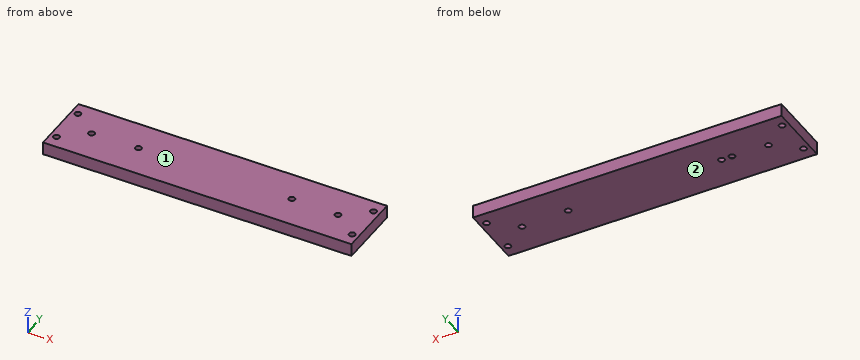
```python
from build123d import *

# Parameters (mm, degrees)
SKETCH1_W                      = 152.4
SKETCH1_H                      = 6.35
WALL_DEPTH                     = 31.75
F_3_0MM_DOWEL_HOLE2_AT_2_COUNT = 2
F_3_0MM_DOWEL_HOLE2_AT_2_PITCH = 19.05
F_3_0MM_DOWEL_HOLE1_D          = 3
F_3_0MM_DOWEL_HOLE1_DEPTH      = 12.7
F_3_0MM_DOWEL_HOLE1_TIP        = 0.901290929
F_3_0MM_DOWEL_HOLE4_D          = 3
F_3_0MM_DOWEL_HOLE4_DEPTH      = 12.7
F_3_0MM_DOWEL_HOLE4_TIP        = 0.901290929
F_3_0MM_DOWEL_HOLE5_OUTLINE_R  = 1.5
F_3_0MM_DOWEL_HOLE5_DEPTH      = 6.35


# Read off the part's stored shape, not the designer's step: Ø3.0mm Dowel Hole5, Ø3.0mm Dowel Hole6
with BuildPart() as part:
    # Sketch1 → wall (new body)
    with BuildSketch(Plane(origin=(0, 0, 0), x_dir=(1, 0, 0), z_dir=(0, 1, 0))):
        with Locations((0, -3.175)):
            Rectangle(SKETCH1_W, SKETCH1_H)
    extrude(amount=WALL_DEPTH)

    # Sketch5 → Ø3.0mm Dowel Hole2 (revolve, cut)
    with BuildSketch(Plane(origin=(-73.025, 25.4, 0), x_dir=(0, 1, 0), z_dir=(1, 0, 0))):
        Polygon((0, 0), (0, 15.901286329), (1.5, 14.9999954), (1.5, 0), align=None)
    f_3_0mm_dowel_hole2 = revolve(axis=Axis((-73.025, 25.4, -6.35), (0, 0, 1)), mode=Mode.SUBTRACT)

    # Ø3.0mm Dowel Hole2 at 2: Ø3.0mm Dowel Hole2 ×2
    with Locations(*[(0, -i * F_3_0MM_DOWEL_HOLE2_AT_2_PITCH, 0) for i in range(1, F_3_0MM_DOWEL_HOLE2_AT_2_COUNT)]):
        add(f_3_0mm_dowel_hole2, mode=Mode.SUBTRACT)

    # Mirror1: Ø3.0mm Dowel Hole2 across plane
    add(f_3_0mm_dowel_hole2.mirror(Plane(origin=(0, 0, 0), x_dir=(0, 0, 1), z_dir=(1, 0, 0))), mode=Mode.SUBTRACT)

    # Mirror1 copy 1 sketch → Mirror1 copy 1 (revolve, cut)
    with BuildSketch(Plane(origin=(73.025, 6.35, 0), x_dir=(0, 1, 0), z_dir=(-1, 0, 0))):
        Polygon((0, 0), (0, -15.901286329), (1.5, -14.9999954), (1.5, 0), align=None)
    revolve(axis=Axis((73.025, 6.35, -6.35), (0, 0, -1)), mode=Mode.SUBTRACT)

    # Ø3.0mm Dowel Hole1
    with Locations(Plane(origin=(76.2, 31.75, -2.54), x_dir=(1, 0, 0), z_dir=(0, 0, -1))):
        with Locations((-137.16, 15.875)):
            Hole(F_3_0MM_DOWEL_HOLE1_D / 2, depth=F_3_0MM_DOWEL_HOLE1_DEPTH)
            with Locations((0, 0, -(F_3_0MM_DOWEL_HOLE1_DEPTH + F_3_0MM_DOWEL_HOLE1_TIP / 2))):  # 118° drill point
                Cone(0, F_3_0MM_DOWEL_HOLE1_D / 2, F_3_0MM_DOWEL_HOLE1_TIP, mode=Mode.SUBTRACT)

    # Ø3.0mm Dowel Hole4
    with Locations(Plane(origin=(76.2, 31.75, -2.54), x_dir=(1, 0, 0), z_dir=(0, 0, -1))):
        with Locations((-38.439194916, 15.502033877), (-15.376273346, 16.029273481)):
            Hole(F_3_0MM_DOWEL_HOLE4_D / 2, depth=F_3_0MM_DOWEL_HOLE4_DEPTH)
            with Locations((0, 0, -(F_3_0MM_DOWEL_HOLE4_DEPTH + F_3_0MM_DOWEL_HOLE4_TIP / 2))):  # 118° drill point
                Cone(0, F_3_0MM_DOWEL_HOLE4_D / 2, F_3_0MM_DOWEL_HOLE4_TIP, mode=Mode.SUBTRACT)

    # Ø3.0mm Dowel Hole5 outline → Ø3.0mm Dowel Hole5 (cut)
    with BuildSketch(Plane.XY):
        with Locations((-38.1, 16.386133576)):
            Circle(F_3_0MM_DOWEL_HOLE5_OUTLINE_R)
    extrude(amount=F_3_0MM_DOWEL_HOLE5_DEPTH, mode=Mode.SUBTRACT)

    # Ø3.0mm Dowel Hole6 outline → Ø3.0mm Dowel Hole6 (revolve, cut)
    with BuildSketch(Plane(origin=(-43.247895679, 16.386133576, 0), x_dir=(1, 0, 0), z_dir=(0, -1, 0))):
        Polygon((1.5, 0.186037407), (0, 1.087328336), (0, 0), (1.5, 0), align=None)
    revolve(axis=Axis((-43.247895679, 16.386133576, 0), (0, 0, 1)), mode=Mode.SUBTRACT)


solid = part.part
```
Can you work these out from the model? Positions are in its coordinate system, mm. Face numbers are marked on the shaded views. Coordinates: 2 decimals unless noted, no trailing zeros. Write each loop counter-clockwise with the first axis right and the second up, starting at its lowest first coordinate (ties: lowest second). Pieces come first, ordered by that corner, then holes. Notation, with made-up numbers: M -8.75,34.5 L 40.25,34.5 A25 ccw 40.25,60.5 Z; hole C -17,6.25 d2. An arc over 180 degrees is marked long. Answer as CSV lines item,"result".
Item 1: Imagine slicing it at B-B on y = 6.35. List the corners of the cut face in (x, z) for me (3 decimals).
Geometry results:
outline,"M -76.2,0 L -74.525,0 L -74.525,6.35 L -76.2,6.35 Z; M -71.525,0 L 71.525,0 L 71.525,6.35 L -71.525,6.35 Z; M 74.525,0 L 76.2,0 L 76.2,6.35 L 74.525,6.35 Z"
Item 2: We'd pull the mould along Z, two halves only. Please class the marked faces 1 and 2: +Z half, -Z half, draft (parallel to the pull), parting line (faces both ways), or undercut.
Geometry results:
face 1,"+Z half"
face 2,"-Z half"
Item 3: Please list where this line runs through material, in increasing order: line 1 along X through (y, z) = (6.5, 2.75).
Geometry results:
line 1,"x = -76.2 to -74.52, -71.53 to 71.53, 74.52 to 76.2"
Item 4: Imagine slicing it at A-A on x = -38.1. List the corners of the cut face in (y, z) for me.
Geometry results:
outline,"M 0,0 L 14.89,0 L 14.89,6.35 L 0,6.35 Z; M 17.89,0 L 31.75,0 L 31.75,6.35 L 17.89,6.35 Z"
